CAD build for the part. Positions are in the model's coordinates, mm. A direction names the side the tool comes from. Round coordinates to 2 decimals unless told otherwise and drop trailing zeros. Loops run counter-clockwise (first coordinate to the right, second up) from the corner with the lowest first, then second, coordinate; pieces in that order, holes last. Notation, with made-up numbers: (58.25, 17) - (106.25, 17) arc R20 ccw to (106.25, 31) - close; hole circle Ø2 at (20.25, 24). An arc over 180 degrees is marked (long way). Use one line per item in the form item = value.
Autodesk Inventor part; units mm, degrees
ref_plane "YZ Plane" through (0, 0, 0) normal (1, 0, 0) x (0, 1, 0)
ref_plane "XZ Plane" through (0, 0, 0) normal (0, 1, 0) x (-1, 0, 0)
ref_plane "XY Plane" through (0, 0, 0) normal (0, 0, 1) x (1, 0, 0)
sketch "Sketch1" plane through (0, 0, 0) normal (0, 0, 1) x (1, 0, 0)
  line L0 (-190, 100) -> (190, 100)
  line L1 (190, 100) -> (190, -100)
  line L2 (190, -100) -> (-190, -100)
  line L3 (-190, -100) -> (-190, 100)
  line L4 (-190, 100) -> (190, -100) construction
  point P0 (0, 0)
  point P1 (0, 0)
  dimension "d0" = 380
  dimension "d1" = 200
extrude "Plate1" add sketch "Sketch1" against normal blind 3
sketch "Sketch2" plane through (0, 0, 0) normal (0, 0, 1) x (1, 0, 0)
  line L0 (60, 56) -> (150, 56) construction
  line L1 (150, 56) -> (150, -56) construction
  line L2 (150, -56) -> (60, -56) construction
  line L3 (60, -56) -> (60, 56) construction
  line L4 (190, -100) -> (190, 100)
  point P0 (0, 0)
  point P1 (60, 0)
  dimension "d3" = 90
  dimension "d4" = 112
  dimension "d5" = 40
hole "Hole1" at (60, 56, 0) at (150, 56, 0) at (60, -56, 0) at (150, -56, 0) direction (0, 0, -1) diameter 12 end through all
sketch "Sketch3" plane through (0, 0, 0) normal (0, 0, 1) x (1, 0, 0)
  line L0 (-175, 85) -> (175, 85) construction
  line L1 (175, 85) -> (175, -85) construction
  line L2 (175, -85) -> (-175, -85) construction
  line L3 (-175, -85) -> (-175, 85) construction
  line L4 (-175, 85) -> (175, -85) construction
  point P0 (0, 0)
  point P1 (0, 0)
  dimension "d14" = 170
  dimension "d15" = 350
hole "Hole2" at (-175, 85, 0) at (175, 85, 0) at (175, -85, 0) at (-175, -85, 0) direction (0, 0, -1) diameter 10 end through all
sketch "Sketch4" plane through (-190, -97, 0) normal (0, -1, 0) x (1, 0, 0)
  line L0 (380, 0) -> (0, 0)
  line L1 (0, 0) -> (0, -25)
  line L2 (0, -25) -> (380, -25)
  line L3 (380, -25) -> (380, 0)
edge flange "Flange1" height 25 angle 90 thickness 3 bend radius 5 thickness toward (0, -1, 0) relief round relief width 3 relief depth 1.5 corner gap 5 corner form 0 edges at (0, -100, -3) (0, 100, -3) wall of the first edge with corners at (190, -97, 0) (-190, -97, 0) (-190, -97, -25) (190, -97, -25)
bend "Bend1"
corner "Corner1"
equation "\"d11\" = Thickness"
equation "\"d2\" = Thickness"
equation "\"d23\" = BendReliefWidth"
equation "\"d24\" = BendReliefDepth"
equation "\"d25\" = MinimumRemnant"
equation "\"d26\" = TransitionRadius"
equation "\"d29\" = BendRadius"
equation "\"d30\" = CornerReliefSize"
equation "\"d31\" = GapSize"
equation "\"d32\" = JacobiRadiusSize"
equation "\"BendReliefWidth\" = Thickness"
equation "\"BendReliefDepth\" = 0.5 * Thickness"
equation "\"CornerReliefSize\" = 4 * Thickness"
equation "\"MinimumRemnant\" = 2 * Thickness"
equation "\"TransitionRadius\" = BendRadius"
equation "\"JacobiRadiusSize\" = BendRadius"
equation "\"GapSize\" = Thickness"
properties part number "BURUN plate" material "Stainless Steel"
1) Two-plate mould, pull along X, no slides. Class faces 3 (the flat face through (-190, 0, -1)), 4 (the flat face through (3, 97, -16)), 5 (the cylindrical face through (-179.957, -84.349, -1.521)): +X half, -X half, draft (parallel to the pull), parting line (faces both ways), or undercut.
Report:
face_3 = -X half
face_4 = draft
face_5 = undercut
2) Drill centre lines: probe 1 along X at (y, z) = (-56, -2); probe 2 along Y at (x, z) = (-15, -8.25); probe 3 along Y at (x, z) = (175, -2.1). Where is each one in solid material? Low to high.
Report:
probe_1 = -190 to 54, 66 to 144, 156 to 190
probe_2 = -100 to -97, 97 to 100
probe_3 = -97.4 to -90, -80 to 80, 90 to 97.4
3) Tool access for faces 1 (the flat face through (-3, 1, -3)), 2 (the cylindrical face through (60, 62, -2)): list every direction of +Z, -Z, +X, -X, +Y, -Y with a clear straight run to the whole face (end or side of a thin tool).
Report:
face_1 = -Z, +X, -X
face_2 = +Z, -Z
4) Slice it at C-C (z = -18). Write the cut outline in (x, y).
Report:
outline = (-190, -100) - (190, -100) - (190, -97) - (-190, -97) - close; (-190, 97) - (190, 97) - (190, 100) - (-190, 100) - close
5) Flat gauge pins, fed straight in: pin 1 (8 mm diameter, centred on x = -96, z = -7.5, fed in from +Y); pin 2 (1.5 mm diameter, centred on x = 55, z = -3.5, fed in from +Y); pin 3 (4 mm diameter, centred on x = -38, y = -48.5, fed in from -Z). Where does each tip first touch, or does it go through?
Report:
pin_1 = 100
pin_2 = 99.07
pin_3 = -3
6) Slice it at A-A (y = -56). Write the cut outline in (x, z), plus the area to 3 significant figures.
Report:
outline = (-190, -3) - (54, -3) - (54, 0) - (-190, 0) - close; (66, -3) - (144, -3) - (144, 0) - (66, 0) - close; (156, -3) - (190, -3) - (190, 0) - (156, 0) - close
area = 1,070 mm^2
7) Slice it at B-B (x = 175). Write the cut outline in (y, z).
Report:
outline = (-100, -25) - (-97, -25) - (-97, -8) arc R5 cw to (-92, -3) - (-90, -3) - (-90, 0) - (-92, 0) arc R8 ccw to (-100, -8) - close; (-80, -3) - (80, -3) - (80, 0) - (-80, 0) - close; (90, -3) - (92, -3) arc R5 cw to (97, -8) - (97, -25) - (100, -25) - (100, -8) arc R8 ccw to (92, 0) - (90, 0) - close
8) Slice it at D-D (x = 132.5). Write the cut outline in (y, z).
Report:
outline = (-100, -25) - (-97, -25) - (-97, -8) arc R5 cw to (-92, -3) - (92, -3) arc R5 cw to (97, -8) - (97, -25) - (100, -25) - (100, -8) arc R8 ccw to (92, 0) - (-92, 0) arc R8 ccw to (-100, -8) - close
